The listing builds one solid part. Answer for the finished solid, in the listing's coordinates (mm). Coordinates: 2 decimals unless noted, no trailing zeros. Write each loop counter-clockwise with the first axis right and the second up, starting at its lowest first coordinate (ties: lowest second). Pieces come first, ordered by that corner, then holes.
(1) Given P1, Ø12, axis at y = -35.5, z = -141, coming from the -X side; P2, Ø8, axis at x = 11.5, y = -25, coming from the -Z side; P3, Ø4, axis at x = 53, z = 220, coming from the +Y side; P4, Ø5, axis at x = -52, z = 179.5, coming from the -Y side, each flat-ended and moving along its own axis, determine where each tip first touches the part or whether it passes through.
(2) The part is cut by section B-B on z = -10. Determine the outline of the cut face in (x, y).
(3) The part is cut by section C-C on x = -44.5. Determine the outline of the cut face in (y, z), plus the area to 3 significant figures.
(4) Straight lines are drawn through the part: line 1 (Z direction, x = -53, y = -45.2); line 2 (X direction, y = -44, z = 220); line 3 (Y direction, x = 41, z = 207). For each, find the intervals that lie inside material, in ascending order.
(5) The part is cut by section A-A on y = -64.5. Determine the outline of the cut face in (x, z).
from build123d import *

# Parameters (mm, degrees)
EXTRUDE_START    = 130
EXTRUDE_1_DEPTH  = 10
EXTRUDE_START_2  = -130
EXTRUDE_2_DEPTH  = 15
SKETCH_2_R       = 3.5
EXTRUDE_5_DEPTH  = 5
EXTRUDE_START_3  = -20
EXTRUDE_11_DEPTH = 20
EXTRUDE_15_DEPTH = 15
EXTRUDE_16_DEPTH = 5
FILLET_1_R       = 10
SKETCH_9_W       = 74.478184726
SKETCH_9_H       = 2
EXTRUDE_17_DEPTH = 30


with BuildPart() as part:
    # Sketch 1 → Extrude 1 (new, symmetric)
    with BuildSketch(Plane.XY.offset(EXTRUDE_START)):
        with BuildLine():
            Line((-34.641016151, -20), (-37.239092363, -21.5))
            ThreePointArc((-37.239092363, -21.5), (0, -43), (37.239092363, -21.5))
            Line((37.239092363, -21.5), (34.641016151, -20))
            ThreePointArc((34.641016151, -20), (0, -40), (-34.641016151, -20))
        make_face()
    extrude(amount=EXTRUDE_1_DEPTH, both=True)



with BuildPart() as body_2:
    # Sketch 1_2 → Extrude 2 (new body)
    with BuildSketch(Plane.XY.offset(EXTRUDE_START_2)):
        with BuildLine():
            Line((-34.641016151, -20), (-37.239092363, -21.5))
            ThreePointArc((-37.239092363, -21.5), (0, -43), (37.239092363, -21.5))
            Line((37.239092363, -21.5), (34.641016151, -20))
            ThreePointArc((34.641016151, -20), (0, -40), (-34.641016151, -20))
        make_face()
    extrude(amount=-EXTRUDE_2_DEPTH)

    # Sketch 7 → Extrude 15 (add)
    with BuildSketch(Plane(origin=(0, 0, -145), x_dir=(-1, 0, 0), z_dir=(0, 0, -1))):
        with BuildLine():
            Line((37.239092363, -21.5), (37.239092363, -48))
            Line((37.239092363, -48), (-37.239092363, -48))
            Line((-37.239092363, -48), (-37.239092363, -21.5))
            ThreePointArc((-37.239092363, -21.5), (0, -43), (37.239092363, -21.5))
        make_face()
    extrude(amount=-EXTRUDE_15_DEPTH)


with BuildPart() as body_3:
    # Sketch 2 → Extrude 5 (new body)
    with BuildSketch(Plane(origin=(0, -43, 0), x_dir=(-1, 0, 0), z_dir=(0, -1, 0))):
        Polygon((-37.239092363, -180), (-68, -180), (-68, -434.984182396), (68, -434.984182396), (68, -180), (37.239092363, -180), (37.239092363, -120), (-37.239092363, -120), align=None)
        with Locations(Location((-53, -220, 0), (0, 0, 90))):
            Circle(SKETCH_2_R, mode=Mode.SUBTRACT)
        with Locations(Location((-53, -420, 0), (0, 0, 90))):
            Circle(SKETCH_2_R, mode=Mode.SUBTRACT)
        with Locations(Location((53, -420, 0), (0, 0, 270))):
            Circle(SKETCH_2_R, mode=Mode.SUBTRACT)
        with Locations(Location((53, -220, 0), (0, 0, 270))):
            Circle(SKETCH_2_R, mode=Mode.SUBTRACT)
    extrude(amount=EXTRUDE_5_DEPTH)


with BuildPart() as part_1:
    add(part.part)

    add(body_3.part)  # Extrude 11 merges body 3
    # Sketch 5 → Extrude 11 (add)
    with BuildSketch(Plane(origin=(0, 0, 120), x_dir=(-1, 0, 0), z_dir=(0, 0, -1)).offset(EXTRUDE_START_3)):
        with BuildLine():
            Line((-37.239092363, -21.5), (-37.239092363, -48))
            Line((-37.239092363, -48), (37.239092363, -48))
            Line((37.239092363, -48), (37.239092363, -21.5))
            ThreePointArc((37.239092363, -21.5), (0, -43), (-37.239092363, -21.5))
        make_face()
    extrude(amount=EXTRUDE_11_DEPTH)


    add(body_2.part)  # Extrude 16 merges body 2
    # Sketch 8 → Extrude 16 (add, symmetric)
    with BuildSketch(Plane(origin=(0, 0, 0), x_dir=(0, 0, -1), z_dir=(1, 0, 0))):
        Polygon((-140, -43), (-140, -120), (145, -120), (145, -43), (130, -43), (130, -48), (130, -110), (-120, -110), (-120, -48), (-120, -43), align=None)
    extrude(amount=EXTRUDE_16_DEPTH, both=True)

    # Fillet 1
    fillet_1_edges = [part_1.edges().sort_by_distance(p)[0] for p in [
        (-5, -48, 130),
        (5, -48, 130),
        (-5, -48, -137.5),
        (5, -48, -137.5),
    ]]
    fillet(fillet_1_edges, radius=FILLET_1_R)

    # Sketch 9 → Extrude 17 (add)
    with BuildSketch(Plane(origin=(0, -43, 0), x_dir=(1, 0, 0), z_dir=(0, 1, 0))):
        with Locations((0, -141)):
            Rectangle(SKETCH_9_W, SKETCH_9_H)
    extrude(amount=EXTRUDE_17_DEPTH)


solid = part_1.part
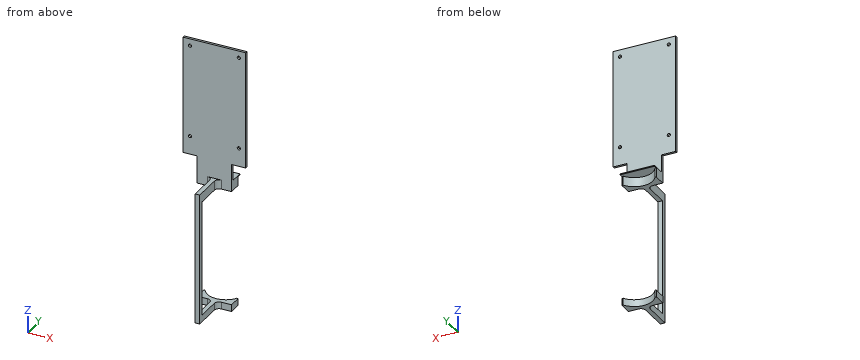
Model answer:
1. P1: stops at x = -37.24
1. P2: stops at z = 140
1. P3: passes through
1. P4: stops at y = -48
2. outline: (-5, -120) - (5, -120) - (5, -110) - (-5, -110) - close
3. outline: (-48, 180) - (-43, 180) - (-43, 434.98) - (-48, 434.98) - close
3. area: 1,270 mm2
4. line 1: z = 180 to 216.5, 223.5 to 416.5, 423.5 to 434.98
4. line 2: x = -68 to -56.5, -49.5 to 49.5, 56.5 to 68
4. line 3: y = -48 to -43
5. outline: (-5, -145) - (5, -145) - (5, -130) - (-5, -130) - close; (-5, 120) - (5, 120) - (5, 140) - (-5, 140) - close
